from build123d import *

# Parameters (mm, degrees)
BOSS_EXTRUDE1_DEPTH = 6.35
SKETCH2_R           = 1.025
SKETCH2_W           = 0.7
SKETCH2_H           = 1.85
CUT_EXTRUDE1_DEPTH  = 6.35


with BuildPart() as part:
    # Sketch1 → Boss-Extrude1 (new body)
    with BuildSketch(Plane(origin=(0, 0, 0), x_dir=(1, 0, 0), z_dir=(0, 1, 0))):
        with BuildLine():
            Line((5, 0), (65, 0))
            ThreePointArc((65, 0), (68.535533906, 1.464466094), (70, 5))
            Line((70, 5), (70, 22.27))
            ThreePointArc((70, 22.27), (68.535533906, 25.805533906), (65, 27.27))
            Line((65, 27.27), (5, 27.27))
            ThreePointArc((5, 27.27), (1.464466094, 25.805533906), (0, 22.27))
            Line((0, 22.27), (0, 5))
            ThreePointArc((0, 5), (1.464466094, 1.464466094), (5, 0))
        make_face()
    extrude(amount=BOSS_EXTRUDE1_DEPTH)

    # Sketch2 → Cut-Extrude1 (cut)
    with BuildSketch(Plane(origin=(0, 6.35, 0), x_dir=(1, 0, 0), z_dir=(0, 1, 0))):
        with Locations(Location((12.5, 13.635, 0), (0, 0, 270))):
            Circle(SKETCH2_R)
        with Locations(Location((17.5, 13.635, 0), (0, 0, 270))):
            Circle(SKETCH2_R)
        with Locations(Location((52.5, 13.635, 0), (0, 0, 270))):
            Circle(SKETCH2_R)
        with Locations(Location((57.5, 13.635, 0), (0, 0, 270))):
            Circle(SKETCH2_R)
        with Locations((15, 15.21)):
            Rectangle(SKETCH2_W, SKETCH2_H)
        with Locations((15, 12.06)):
            Rectangle(SKETCH2_W, SKETCH2_H)
        with Locations((55, 12.06)):
            Rectangle(SKETCH2_W, SKETCH2_H)
        with Locations((55, 15.21)):
            Rectangle(SKETCH2_W, SKETCH2_H)
    extrude(amount=-CUT_EXTRUDE1_DEPTH, mode=Mode.SUBTRACT)


solid = part.part
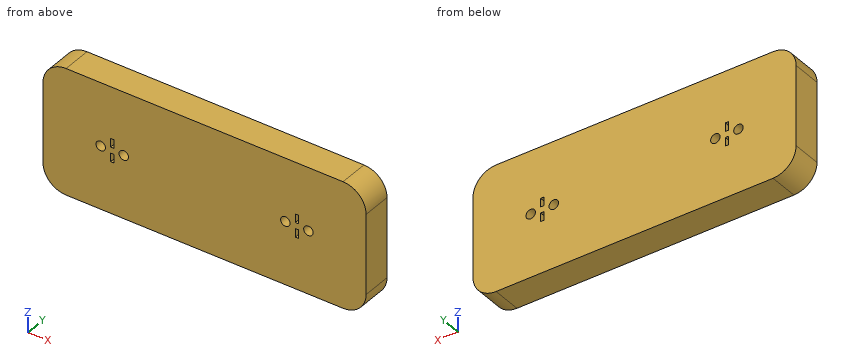
Work out the finished part from the listing and answer in its coordinate system (mm). Give positions to 0.01 mm unless a question says otherwise; leave off trailing zeros. Write each loop counter-clockwise with the first axis right and the second up, starting at its lowest first coordinate (ties: lowest second). Pieces come first, ordered by that corner, then holes.
Q1. The part is cut by section B-B on y = 5.5. State how many separate pieces and enclosed holes the cut face has, and give its area (3 significant figures).
Answer:
separate pieces: 1
enclosed holes: 8
area: 1,870 mm2
Q2. Straight lines are drawn through the part: L1, parallel to X at y = 1.25, z = -15.25; L2, parallel to Z at x = 55, y = 2 (3 decimals); L3, parallel to X at y = 5.5, z = -4.75. For each, find the intervals that lie inside material, in ascending order.
Answer:
L1: x = 0 to 14.65, 15.35 to 54.65, 55.35 to 70
L2: z = -27.27 to -16.135, -14.285 to -12.985, -11.135 to 0
L3: x = 0.01 to 69.99
Q3. The part is cut by section A-A on x = 17.5. Give the vertices of the cut face in (y, z), and give its area (3 significant figures).
Answer:
outline: (0, -27.27) - (6.35, -27.27) - (6.35, -14.66) - (0, -14.66) - close; (0, -12.61) - (6.35, -12.61) - (6.35, 0) - (0, 0) - close
area: 160 mm2
Q4. Given pin 1 (2.5 mm diameter, centred on x = 57.5, z = -13.635, fed in from +Y); pin 2 (1.6 mm diameter, centred on x = 12.5, z = -13.635, fed in from +Y), each flat-ended and moving along its own axis, determine where each tip first touches the part or whether it passes through.
Answer:
pin 1: stops at y = 6.35
pin 2: passes through
